Build history of the part. All positions in model axes, mm. Face numbers are marked on the shaded views. A direction names the side the tool comes from. Round coordinates to 2 decimals unless told otherwise and drop trailing zeros. Write each loop counter-clockwise with the first axis right and the second up, starting at its lowest first coordinate (ties: lowest second). Pieces come first, ordered by that corner, then holes. Notation, with made-up numbers: (54, 69) - (97, 69) arc R6 cw to (97, 78) - close; hole circle Ø3 at (59.5, 24). An arc over 180 degrees is marked (long way). Write each question's results on one line, items separated by ' | '.
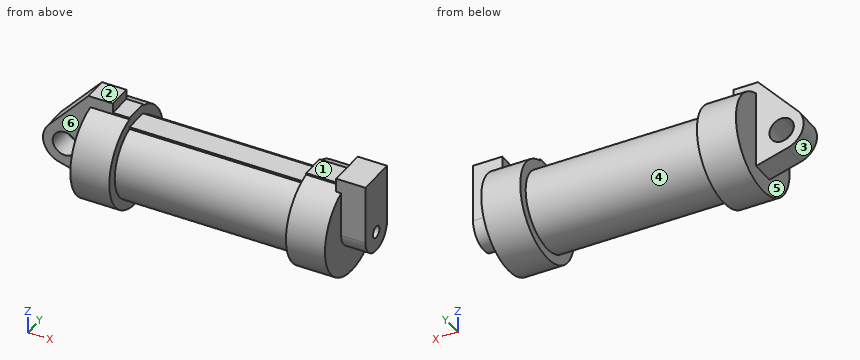
from build123d import *

# Parameters (mm, degrees)
F0_W          = 5.842
F0_H          = 12.7
F0_R          = 3.175
F2_DEPTH      = 3.175
F3_R          = 1.524
F4_DEPTH      = 1.27
F4_DEPTH_BACK = 6.35


with BuildPart() as f1:
    # F0 (on Front) → F1 (revolve)
    with BuildSketch(Plane.XZ):
        Polygon((5.842, 12.7), (5.842, 0), (66.294, 0), (66.294, 12.7), (56.134, 12.7), (56.134, 10.16), (10.16, 10.16), (10.16, 12.7), align=None)
        with Locations((2.921, 6.35)):
            Rectangle(F0_W, F0_H)
    revolve(axis=Axis((33.147, 0, 0), (-1, 0, 0)))

    # F0 (on Front) → F2 (join, symmetric)
    with BuildSketch(Plane.XZ):
        Polygon((5.842, 12.7), (5.842, 0), (66.294, 0), (66.294, 12.7), (56.134, 12.7), (56.134, 10.16), (10.16, 10.16), (10.16, 12.7), align=None)
        with Locations((2.921, 6.35)):
            Rectangle(F0_W, F0_H)
        with BuildLine():
            Line((-0.9398, 0), (0, 0))
            Line((0, 0), (0, 12.7))
            Line((0, 12.7), (5.842, 12.7))
            Line((5.842, 12.7), (5.842, 15.24))
            Line((5.842, 15.24), (-0.508, 15.24))
            Line((-0.508, 15.24), (-10.8806298187, 3.8475430269))
            ThreePointArc((-10.8806298187, 3.8475430269), (-4.5919612295, 5.3297205562), (-0.9398, 0))
        make_face()
        with BuildLine():
            Line((5.842, 0), (0, 0))
            Line((0, 0), (-0.9398, 0))
            ThreePointArc((-0.9398, 0), (-3.1957909266, -4.5493385486), (-8.1826630726, -5.5069827884))
            Line((-8.1826630726, -5.5069827884), (5.842, -9.398))
            Line((5.842, -9.398), (5.842, 0))
        make_face()
        with BuildLine():
            ThreePointArc((-8.1826630726, -5.5069827884), (-3.1957909266, -4.5493385486), (-0.9398, 0))
            ThreePointArc((-0.9398, 0), (-4.5919612295, 5.3297205562), (-10.8806298187, 3.8475430269))
            ThreePointArc((-10.8806298187, 3.8475430269), (-12.1459778134, -1.5837270034), (-8.1826630726, -5.5069827884))
        make_face()
        with Locations((-6.6548, 0)):
            Circle(F0_R, mode=Mode.SUBTRACT)
    extrude(amount=F2_DEPTH, both=True)

    # F3 (on face) → F4 (join, two sides)
    with BuildSketch(Plane.YZ.offset(66.294)) as f4_sk:
        with BuildLine():
            ThreePointArc((-5.08, 0), (0, -5.08), (5.08, 0))
            ThreePointArc((5.08, 0), (0, 5.08), (-5.08, 0))
        make_face()
        Circle(F3_R, mode=Mode.SUBTRACT)
        with BuildLine():
            ThreePointArc((-5.08, 0), (0, 5.08), (5.08, 0))
            Line((5.08, 0), (5.08, 15.24))
            Line((5.08, 15.24), (-5.08, 15.24))
            Line((-5.08, 15.24), (-5.08, 0))
        make_face()
    extrude(amount=-F4_DEPTH)
    extrude(f4_sk.sketch, amount=F4_DEPTH_BACK)


solid = f1.part
(1) Two-plate mould, pull along X, no slides. Class the marked faces 1, 2 and 3: released by +X, released by -X, zero draft, split by the parting line, or undercut.
Worked answers:
face 1: undercut | face 2: zero draft | face 3: released by -X
(2) Drill centre lines: probe 1 along X at (y, z) = (-10, -6.25); probe 2 along X at (y, z) = (8.5, -5); probe 3 along Y at (x, z) = (-4.5, 5.75) (3 decimals). Where is each one in solid material? Low to high. Write a range as [from, to].
Worked answers:
probe 1: x = [0, 10.16], [56.13, 66.29] | probe 2: x = [0, 66.29] | probe 3: y = [-3.175, 3.175]
(3) Slice it at A-A, the plane y = 0. Write the cut outline in (x, z) (3 decimals).
Worked answers:
outline: (-10.881, 3.848) arc R5.715 ccw to (-8.183, -5.507) - (0, -7.777) - (0, -12.7) - (10.16, -12.7) - (10.16, -10.16) - (56.134, -10.16) - (56.134, -12.7) - (66.294, -12.7) - (66.294, -5.08) - (72.644, -5.08) - (72.644, -1.524) - (66.294, -1.524) - (66.294, 1.524) - (72.644, 1.524) - (72.644, 15.24) - (65.024, 15.24) - (65.024, 12.7) - (56.134, 12.7) - (56.134, 10.16) - (10.16, 10.16) - (10.16, 12.7) - (5.842, 12.7) - (5.842, 15.24) - (-0.508, 15.24) - close; hole circle Ø6.35 at (-6.655, 0)
(4) Slice it at B-B, the plane x = 49. Write the cut outline in (y, z) (3 decimals).
Worked answers:
outline: (-3.175, 9.651) arc R10.16 ccw (long way) to (3.175, 9.651) - (3.175, 10.16) - (-3.175, 10.16) - close
(5) Slice it at C-C, the plane z = 7.75. Write the cut outline in (x, y) (3 decimals).
Worked answers:
outline: (-7.328, -3.175) - (0, -3.175) - (0, -10.061) - (10.16, -10.061) - (10.16, -6.57) - (56.134, -6.57) - (56.134, -10.061) - (66.294, -10.061) - (66.294, -5.08) - (72.644, -5.08) - (72.644, 5.08) - (66.294, 5.08) - (66.294, 10.061) - (56.134, 10.061) - (56.134, 6.57) - (10.16, 6.57) - (10.16, 10.061) - (0, 10.061) - (0, 3.175) - (-7.328, 3.175) - close
(6) Slice it at D-D, the plane x = 4. Write the cut outline in (y, z) (3 decimals), and give its area (3 significant figures).
Worked answers:
outline: (-3.175, 12.297) arc R12.7 ccw (long way) to (3.175, 12.297) - (3.175, 15.24) - (-3.175, 15.24) - close | area: 524 mm2
(7) Tool access for the marked faces 4, 5 and 6: list every direction of +Z, -Z, +X, -X, +Y, -Y with a clear straight run to the whole face (end or side of a thin tool).
Worked answers:
face 4: none | face 5: -Z, -X | face 6: +Z, -X, -Y
(8) Flat gauge pins, fed straight in: pin 1 Ø1.9 at (x, y) = (60, 0.5) entering from +Z; pin 2 Ø4 at (y, z) = (0.5, 13) entering from -X; pin 3 Ø8 at (x, y) = (49, -8) entering from +Z. Where does each tip first touch, or does it go through?
Worked answers:
pin 1: stops at z = 12.7 | pin 2: stops at x = -4.37 | pin 3: stops at z = 9.34
